Solid Edge part; units mm, degrees
sketch "Sketch1" plane through (0, 0, 0) normal (0, 0, 1) x (1, 0, 0)
  line L0 (12.5, 0) -> (12.5, 50)
  line L1 (12.5, 50) -> (25, 50)
  line L2 (25, 50) -> (25, 43)
  line L3 (25, 43) -> (19, 43)
  line L4 (19, 43) -> (19, 36)
  line L5 (19, 36) -> (17.5, 36)
  line L6 (17.5, 36) -> (17.5, 14)
  line L7 (17.5, 14) -> (19, 14)
  line L8 (19, 14) -> (19, 7)
  line L9 (19, 7) -> (25, 7)
  line L10 (25, 7) -> (25, 0)
  line L11 (25, 0) -> (12.5, 0)
  dimension "D1" = 12.5
  dimension "D2" = 25
  dimension "D3" = 19
  dimension "D4" = 19
  dimension "D5" = 25
  dimension "D6" = 17.5
revolve "RevolvedProtrusion1" add sketch "Sketch1" angle 180 about axis through (0, 54, 0) along (0, -1, 0)
CAD build for the part. Positions are in the model's coordinates, mm. A direction names the side the tool comes from. Coordinates: 2 decimals unless noted, no trailing zeros. Write each loop counter-clockwise with the first axis right and the second up, starting at its lowest first coordinate (ties: lowest second). Pieces come first, ordered by that corner, then holes.
(1) Cut at B-B, the plane z = 8.5. List the corners of the cut face in (x, y).
(2) Flat gauge pins, fed straight in: pin 1 (5 mm diameter, centred on y = 40, z = 18, fed in from -X); pin 2 (1.5 mm diameter, centred on x = -3, y = 15, fed in from -Z); pin 3 (15 mm diameter, centred on x = -6.5, z = 10.5, fed in from +Y); pin 4 (2 mm diameter, centred on y = 10, z = 5, fed in from -X). Where does each tip first touch, or does it go through?
(3) Cut at C-C, the plane x = 0. List the corners of the cut face in (y, z), and give its area (3 significant figures).
(4) Cut at D-D, the plane y = 41. List the corners of the cut face in (x, z), and give its area (3 significant figures).
(5) Two-plate mould, pull along Y, no slides. Class faces 3 (the face through (-17, 25, 0)), 4 (the face through (0, 36, 18)), 5 (the face through (0, 50, 13)), 6 (the face through (0.385, 24.846, 17.496)): +Y half, -Y half, draft (parallel to the pull), parting line (faces both ways), or undercut.
(6) Cut at A-A, the plane x = 20.5. List the corners of the cut face in (y, z), and give its area (3 significant figures).
(7) Drill centre lines: probe 1 along Y at (x, z) = (-3, 23); probe 2 along Z at (x, y) = (0, 9); probe 3 along X at (y, z) = (31, 7.5). Where is each one in solid material? Low to high.
(8) 3-axis set-ups, long thin cutter, end or side, ignore diameter. For faces 1 (the face through (0.55, 3.451, 24.994)), 2 (the face through (-2, 7, 20)): which of +Z, -Z, +X, -X, +Y, -Y reach the whole face in a straight line?
Geometry says:
1. outline: (-23.51, 0) - (-9.17, 0) - (-9.17, 50) - (-23.51, 50) - (-23.51, 43) - (-16.99, 43) - (-16.99, 36) - (-15.3, 36) - (-15.3, 14) - (-16.99, 14) - (-16.99, 7) - (-23.51, 7) - close; (9.17, 0) - (23.51, 0) - (23.51, 7) - (16.99, 7) - (16.99, 14) - (15.3, 14) - (15.3, 36) - (16.99, 36) - (16.99, 43) - (23.51, 43) - (23.51, 50) - (9.17, 50) - close
2. pin 1: stops at x = -10.99
2. pin 2: stops at z = 11.92
2. pin 3: stops at y = 50
2. pin 4: stops at x = -18.57
3. outline: (0, 12.5) - (50, 12.5) - (50, 25) - (43, 25) - (43, 19) - (36, 19) - (36, 17.5) - (14, 17.5) - (14, 19) - (7, 19) - (7, 25) - (0, 25) - close
3. area: 376 mm2
4. outline: (-19, 0) - (-12.5, 0) arc R12.5 cw to (12.5, 0) - (19, 0) arc R19 ccw to start
4. area: 322 mm2
5. face 3: draft
5. face 4: undercut
5. face 5: +Y half
5. face 6: undercut
6. outline: (0, 0) - (7, 0) - (7, 14.31) - (0, 14.31) - close; (43, 0) - (50, 0) - (50, 14.31) - (43, 14.31) - close
6. area: 200 mm2
7. probe 1: y = 0 to 7, 43 to 50
7. probe 2: z = 12.5 to 19
7. probe 3: x = -15.81 to -10, 10 to 15.81
8. face 1: +Z, +Y, -Y
8. face 2: +Z
